from build123d import *

# Parameters (mm, degrees)
F1_DEPTH  = 155
F3_DEPTH  = 370
F5_DEPTH  = 50
F6_R      = 6.25
F7_DEPTH  = 25
F8_R      = 3
F9_DEPTH  = 25
F11_DEPTH = 97.5
F13_DEPTH = 75


# Not quite as in the source:
# - a feature names something its author has since deleted; it is built from what else it names


with BuildPart() as f1:
    # F0 (on Front) → F1 (new body, symmetric)
    with BuildSketch(Plane.XZ):
        Polygon((40, -20), (40, 20), (-40, 20), (-40, -20), (-35, -20), (-35, 15), (35, 15), (35, -20), align=None)
    extrude(amount=F1_DEPTH, both=True)

    # F2 (on face) → F3 (join)
    with BuildSketch(Plane.XY.offset(20)):
        Polygon((-40, 145), (-63, 145), (-63, 142), (-43, 142), (-43, 97.9865193367), (-63, 97.9865193367), (-63, 95), (-43, 95), (-40, 95), align=None)
        Polygon((-40, -145), (-40, -95), (-43, -95), (-63, -95), (-63, -97.9865193367), (-43, -97.9865193367), (-43, -142), (-63, -142), (-63, -145), align=None)
        Polygon((43, -95), (40, -95), (40, -145), (63, -145), (63, -142), (43, -142), (43, -97.9865193367), (63, -97.9865193367), (63, -95), align=None)
        Polygon((63, 145), (40, 145), (40, 95), (43, 95), (63, 95), (63, 97.9865193367), (43, 97.9865193367), (43, 142), (63, 142), align=None)
    extrude(amount=-F3_DEPTH)

    # F4 (on Right) → F5 (cut, symmetric)
    with BuildSketch(Plane.YZ):
        with BuildLine():
            Line((114.5, -320), (114.5, -335))
            ThreePointArc((114.5, -335), (120, -340.5), (125.5, -335))
            Line((125.5, -335), (125.5, -320))
            ThreePointArc((125.5, -320), (120, -314.5), (114.5, -320))
        make_face()
        with BuildLine():
            Line((-114.5, -335), (-114.5, -320))
            ThreePointArc((-114.5, -320), (-120, -314.5), (-125.5, -320))
            Line((-125.5, -320), (-125.5, -335))
            ThreePointArc((-125.5, -335), (-120, -340.5), (-114.5, -335))
        make_face()
    extrude(amount=F5_DEPTH, both=True, mode=Mode.SUBTRACT)

    # F6 (on face) → F7 (cut)
    with BuildSketch(Plane.XY.offset(20)):
        with Locations((0, 45)):
            Circle(F6_R)
        with Locations((0, -45)):
            Circle(F6_R)
    extrude(amount=-F7_DEPTH, mode=Mode.SUBTRACT)

    # F8 (on face) → F9 (cut)
    with BuildSketch(Plane.XY.offset(20)):
        with Locations((-14, 145)):
            Circle(F8_R)
        with Locations((14, 145)):
            Circle(F8_R)
        with Locations((-14, 68)):
            Circle(F8_R)
        with Locations((14, 68)):
            Circle(F8_R)
        with Locations((-14, -68)):
            Circle(F8_R)
        with Locations((14, -68)):
            Circle(F8_R)
        with Locations((-14, -145)):
            Circle(F8_R)
        with Locations((14, -145)):
            Circle(F8_R)
    extrude(amount=-F9_DEPTH, mode=Mode.SUBTRACT)

    # F10 (on Front) → F11 (join, symmetric)
    with BuildSketch(Plane.XZ):
        Polygon((-40, -180), (-63, -180), (-63, -230), (-40, -230), (-40, -227), (-60, -227), (-60, -183), (-40, -183), align=None)
        Polygon((63, -180), (40, -180), (40, -183), (60, -183), (60, -227), (40, -227), (40, -230), (63, -230), align=None)
    extrude(amount=F11_DEPTH, both=True)

    # F12 (on Right) → F13 (cut, symmetric)
    with BuildSketch(Plane.YZ):
        with BuildLine():
            Line((19.9865193367, -200.5), (79.9865193367, -200.5))
            ThreePointArc((79.9865193367, -200.5), (85.4865193367, -195), (79.9865193367, -189.5))
            Line((79.9865193367, -189.5), (19.9865193367, -189.5))
            ThreePointArc((19.9865193367, -189.5), (14.4865193367, -195), (19.9865193367, -200.5))
        make_face()
        with BuildLine():
            ThreePointArc((-79.9865193367, -189.5), (-85.4865193367, -195), (-79.9865193367, -200.5))
            Line((-79.9865193367, -200.5), (-19.9865193367, -200.5))
            ThreePointArc((-19.9865193367, -200.5), (-14.4865193367, -195), (-19.9865193367, -189.5))
            Line((-19.9865193367, -189.5), (-79.9865193367, -189.5))
        make_face()
    extrude(amount=F13_DEPTH, both=True, mode=Mode.SUBTRACT)


solid = f1.part
Can you work these out from the model? Positions are in its coordinate system, mm. A direction names the side the tool comes from. Coordinates: 2 decimals unless noted, no trailing zeros. Loops run counter-clockwise (first coordinate to the right, second up) from the corner with the lowest first, then second, coordinate; pieces in that order, holes last. Notation, with made-up numbers: (-39.75, 30.5) - (-15.75, 30.5) arc R17 ccw to (-15.75, 46.5) - close; hole circle Ø9 at (61, 4.5). An arc over 180 degrees is marked (long way). Put each result on its own line as item: value. Start each with the question number.
Item 1: Suppose I cut it at D-D (x = 0). Please give me the cut outline in (y, z).
Item 2: Suppose I cut it at C-C (z = -50.5). State how many separate pieces and enclosed holes the cut face has, and give its area (3 significant figures).
Item 3: If I drill on line 1 along Y through (x, z) = (0, 17); line 2 along Y through (x, z) = (-14, 17.8); line 3 along Z through (x, y) = (43.5, -1), over which ranges is the centre line in solid material (lowest first)?
Item 4: If we mould it in two halves opening along X, with no side actions, what happens to faces 1 (the face through (-60, 1, -210)), 2 (the face through (40, 150, 0)), 3 (the face through (52, -95, -79))? For each: +X half, -X half, draft (parallel to the pull), parting line (faces both ways), or undercut.
Item 5: Suppose I cut it at B-B (x = 50). Please give me the cut outline in (y, z).
Item 6: Which directions (+Z, -Z, +X, -X, +Y, -Y) give clear straight access to the entire face, cutting with the end or side of a thin tool? Please do faces 4 (the face through (51, 95, -289)), 5 (the face through (-53, -142, -162)), 6 (the face through (-51, -95, -79)).
Item 7: For pin 1 (11.5 mm diameter, centred on x = -56, y = -46, fed in from +Z); pin 2 (22 mm diameter, centred on x = 55, z = -209.5, fed in from +Y); pin 3 (3.5 mm diameter, centred on x = -62, y = -50.5, fed in from -Z), each with a flat end and sliding along its axis, tell me the tip position at first contact or that it passes through.
Item 8: Suppose I cut it at A-A (y = -120). Please give me the cut outline in (x, z), and give its area (3 significant figures).
Here are the results:
1. outline: (-155, 15) - (-51.25, 15) - (-51.25, 20) - (-155, 20) - close; (-38.75, 15) - (38.75, 15) - (38.75, 20) - (-38.75, 20) - close; (51.25, 15) - (155, 15) - (155, 20) - (51.25, 20) - close
2. separate pieces: 4
2. enclosed holes: 0
2. area: 1,080 mm²
3. line 1: -155 to -51.25, -38.75 to 38.75, 51.25 to 155
3. line 2: -155 to -148, -142 to -71, -65 to 65, 71 to 142, 148 to 155
3. line 3: -230 to -227, -183 to -180
4. face 1: undercut
4. face 2: +X half
4. face 3: draft
5. outline: (-145, -350) - (-142, -350) - (-142, 20) - (-145, 20) - close; (-97.99, -350) - (-95, -350) - (-95, -230) - (95, -230) - (95, -350) - (97.99, -350) - (97.99, 20) - (95, 20) - (95, -180) - (-95, -180) - (-95, 20) - (-97.99, 20) - close; (142, -350) - (145, -350) - (145, 20) - (142, 20) - close; hole (-95, -227) - (95, -227) - (95, -183) - (-95, -183) - close
6. face 4: -Z, +X, -X
6. face 5: +Z, -Z, -X
6. face 6: +Z, -X
7. pin 1: z = -180
7. pin 2: y = 145
7. pin 3: z = -230
8. outline: (-43, -350) - (-40, -350) - (-40, -340.5) - (-43, -340.5) - close; (-43, -314.5) - (-40, -314.5) - (-40, -20) - (-35, -20) - (-35, 15) - (35, 15) - (35, -20) - (40, -20) - (40, -314.5) - (43, -314.5) - (43, 20) - (-43, 20) - close; (40, -350) - (43, -350) - (43, -340.5) - (40, -340.5) - close
8. area: 2,810 mm²
